Read the model definition and answer for the solid it produces. Units are mm, in the model's axes. A direction names the side the tool comes from. Give positions to 0.01 mm unless a question says otherwise; leave off trailing zeros. Write each loop counter-clockwise with the first axis right and the second up, starting at its lowest first coordinate (ties: lowest second). Pieces come first, ordered by that corner, then holes. Notation, with made-up numbers: (0, 72) -> (30, 72) arc R13 ccw to (30, 92) -> close; hole circle Ø9 at (-1, -18). An arc over 180 degrees is marked (long way). Use a Markdown table: item, result.
from build123d import *

# Parameters (mm, degrees)
SKETCH1_R           = 1.5
BOSS_EXTRUDE2_DEPTH = 4


with BuildPart() as part:
    # Sketch1 → Boss-Extrude2 (new body)
    with BuildSketch(Plane(origin=(0, 0, 0), x_dir=(1, 0, 0), z_dir=(0, 1, 0))):
        Polygon((-30.100505063, -50), (30.100505063, -50), (47.171572875, -57.071067812), (57.142268085, -67.041763021), (67.041763021, -57.142268085), (57.071067812, -47.171572875), (50, -30.100505063), (50, 30.100505063), (57.071067812, 47.171572875), (67.041763021, 57.142268085), (57.142268085, 67.041763021), (47.171572875, 57.071067812), (30.100505063, 50), (-30.100505063, 50), (-47.171572875, 57.071067812), (-57.142268085, 67.041763021), (-67.041763021, 57.142268085), (-57.071067812, 47.171572875), (-50, 30.100505063), (-50, -30.100505063), (-57.071067812, -47.171572875), (-67.041763021, -57.142268085), (-57.142268085, -67.041763021), (-47.171572875, -57.071067812), align=None)
        with Locations(Location((-57.106667948, -57.106667948, 0), (0, 0, 270))):
            Circle(SKETCH1_R, mode=Mode.SUBTRACT)
        with Locations(Location((-57.106667948, 57.106667948, 0), (0, 0, 90))):
            Circle(SKETCH1_R, mode=Mode.SUBTRACT)
        with Locations(Location((57.106667948, -57.106667948, 0), (0, 0, 90))):
            Circle(SKETCH1_R, mode=Mode.SUBTRACT)
        with Locations(Location((57.106667948, 57.106667948, 0), (0, 0, 270))):
            Circle(SKETCH1_R, mode=Mode.SUBTRACT)
    extrude(amount=BOSS_EXTRUDE2_DEPTH)


solid = part.part
Item 1: A cutting plane is placed at A-A (z = -52). Give the vertices of the cut face in (x, y), then the cut area to 3 significant figures.
Return value:
| item | result |
|---|---|
| outline | (-61.9, 0) -> (-34.93, 0) -> (-34.93, 4) -> (-61.9, 4) -> close; (34.93, 0) -> (61.9, 0) -> (61.9, 4) -> (34.93, 4) -> close |
| area | 216 mm^2 |
Item 2: A tool of negligible diameter and unlimited length cuts with its end or side. For faces 1 (the face through (-53.486, 1.972, 38.517)), 2 (the face through (38.756, 1.972, -53.585)), 3 (the face through (-38.756, 1.972, 53.585)), 4 (the face through (50, 2, 0)), from which of +Z, -Z, +X, -X, +Y, -Y can it reach the whole face along a straight path? Write none if from no direction.
Return value:
| item | result |
|---|---|
| face 1 | -X, +Y, -Y |
| face 2 | -Z, +Y, -Y |
| face 3 | +Z, +Y, -Y |
| face 4 | +X, +Y, -Y |
Item 3: A cutting plane is placed at D-D (z = 18). Give the vertices of the cut face in (x, y), then the cut area to 3 significant figures.
Return value:
| item | result |
|---|---|
| outline | (-50, 0) -> (50, 0) -> (50, 4) -> (-50, 4) -> close |
| area | 400 mm^2 |
Item 4: Each of these flat-tipped pins is pushed along its axis until it touches: P1, Ø2.5, axis at x = 57.11, z = 57.11, coming from the -Y side; P2, Ø1, axis at y = 2.5, z = -48.5, coming from the -X side; P3, Ø2, axis at y = 3, z = -50.5, coming from the +X side; P4, Ø1, axis at x = -21.5, y = 2, coming from the -Z side. Where does it stop, or does it pass through?
Return value:
| item | result |
|---|---|
| P1 | through |
| P2 | x = -58.9 |
| P3 | x = 61.4 |
| P4 | z = -50 |
Item 5: A cutting plane is placed at B-B (x = -52.5). Give the vertices of the cut face in (y, z).
Return value:
| item | result |
|---|---|
| outline | (0, -62.4) -> (4, -62.4) -> (4, -36.14) -> (0, -36.14) -> close; (0, 36.14) -> (4, 36.14) -> (4, 62.4) -> (0, 62.4) -> close |
Item 6: Straight lines are drawn through the part: line 1 along X through (y, z) = (2.15, -4); line 2 along X through (y, z) = (0.5, 61.5). For each, find the intervals that lie inside material, in ascending order. Write a range as [from, to].
Return value:
| item | result |
|---|---|
| line 1 | [-50, 50] |
| line 2 | [-62.68, -51.6], [51.6, 62.68] |
Item 7: A cutting plane is placed at C-C (y = 2.9). Give the vertices of the cut face in (x, z), then the cut area to 3 significant figures.
Return value:
| item | result |
|---|---|
| outline | (-67.04, -57.14) -> (-57.14, -67.04) -> (-47.17, -57.07) -> (-30.1, -50) -> (30.1, -50) -> (47.17, -57.07) -> (57.14, -67.04) -> (67.04, -57.14) -> (57.07, -47.17) -> (50, -30.1) -> (50, 30.1) -> (57.07, 47.17) -> (67.04, 57.14) -> (57.14, 67.04) -> (47.17, 57.07) -> (30.1, 50) -> (-30.1, 50) -> (-47.17, 57.07) -> (-57.14, 67.04) -> (-67.04, 57.14) -> (-57.07, 47.17) -> (-50, 30.1) -> (-50, -30.1) -> (-57.07, -47.17) -> close; hole circle Ø3 at (-57.11, -57.11); hole circle Ø3 at (-57.11, 57.11); hole circle Ø3 at (57.11, -57.11); hole circle Ø3 at (57.11, 57.11) |
| area | 11,400 mm^2 |
Item 8: For a pull along X with two mould halves and no side action, classify faces 5 (the face through (-62.023, 1.972, -62.161)), 6 (the face through (0, 2, 50)), 7 (the face through (53.486, 1.972, -38.517)), 8 (the face through (-1, 4, -1)) as +X half, -X half, draft (parallel to the pull), parting line (faces both ways), or undercut.
Return value:
| item | result |
|---|---|
| face 5 | -X half |
| face 6 | undercut |
| face 7 | +X half |
| face 8 | draft |
